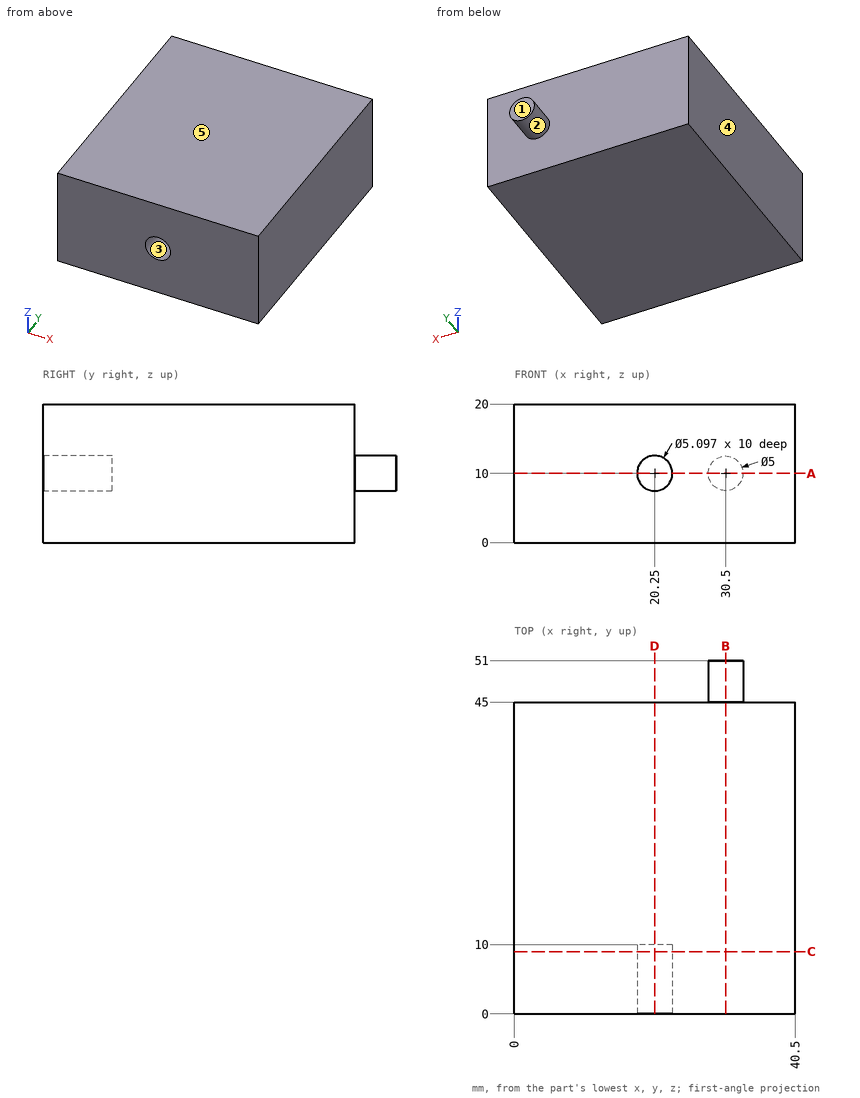
Part print with two shaded views. Sizes in mm from the minimum x, y, z corner. A direction names the side the tool comes from. Round coordinates to 2 decimals unless told otherwise and drop trailing zeros. Write each loop counter-clockwise with the first axis right and the second up, starting at its lowest first coordinate (ties: lowest second). Pieces come first, ordered by that corner, then holes. Notation, with made-up numbers: (-8.5, 87) - (30.5, 87) arc R24 cw to (30.5, 120) - close; hole circle Ø6 at (-26, -8). An arc over 180 degrees is marked (long way). Answer as CSV lines item,"result".
Q1. Cut at B-B (x = 30.5). Write the cut outline in (y, z), and give its area (3 significant figures).
Report:
outline,"(0, 0) - (45, 0) - (45, 7.5) - (51, 7.5) - (51, 12.5) - (45, 12.5) - (45, 20) - (0, 20) - close"
area,"930 mm^2"
Q2. Cut at A-A (z = 10). Write the cut outline in (x, y).
Report:
outline,"(0, 0) - (17.7, 0) - (17.7, 10) - (22.8, 10) - (22.8, 0) - (40.5, 0) - (40.5, 45) - (33, 45) - (33, 51) - (28, 51) - (28, 45) - (0, 45) - close"
Q3. Tool access for the marked faces 1 and 2: list every direction of +Z, -Z, +X, -X, +Y, -Y with a clear straight run to the whole face (end or side of a thin tool).
Report:
face 1,"+Z, -Z, +X, -X, +Y"
face 2,"+Y"
Q4. Cut at D-D (x = 20.25). Write the cut outline in (y, z), and give its area (3 significant figures).
Report:
outline,"(0, 0) - (45, 0) - (45, 20) - (0, 20) - (0, 12.55) - (10, 12.55) - (10, 7.45) - (0, 7.45) - close"
area,"849 mm^2"
Q5. Cut at C-C (y = 9). Write the cut outline in (x, z).
Report:
outline,"(0, 0) - (40.5, 0) - (40.5, 20) - (0, 20) - close; hole circle Ø5.1 at (20.25, 10)"
Q6. Drill centre lines: probe 1 along X at (y, z) = (6.5, 10); probe 2 along Z at (x, y) = (20, 8); probe 3 along Y at (x, z) = (28, 1.5). Where is each one in solid material? Low to high. Write a range as [from, to].
Report:
probe 1,"x = [0, 17.7], [22.8, 40.5]"
probe 2,"z = [0, 7.46], [12.54, 20]"
probe 3,"y = [0, 45]"
Q7. Pull direction Z, two halves, no side cores. Call the marked faces 3, 4 and 5: +Z half, -Z half, draft (parallel to the pull), parting line (faces both ways), or undercut.
Report:
face 3,"undercut"
face 4,"draft"
face 5,"+Z half"
Q8. Drop flat-ended pins along their axis: pin 1 (4 mm diameter, centred on y = 13, z = 17, fed in from -X); pin 2 (6 mm diameter, centred on x = 20.25, z = 10, fed in from +Y); pin 3 (1.5 mm diameter, centred on x = 21, z = 9.5, fed in from -Y). Give the stop position or say it passes through.
Report:
pin 1,"stops at x = 0"
pin 2,"stops at y = 45"
pin 3,"stops at y = 10"
